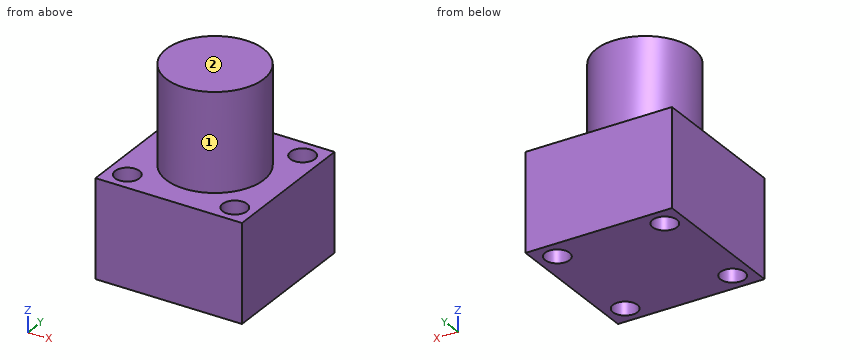
Autodesk Inventor part; units mm, degrees
ref_plane "YZ Plane" through (0, 0, 0) normal (1, 0, 0) x (0, 1, 0)
ref_plane "XZ Plane" through (0, 0, 0) normal (0, 1, 0) x (-1, 0, 0)
ref_plane "XY Plane" through (0, 0, 0) normal (0, 0, 1) x (1, 0, 0)
sketch "Sketch1" plane through (0, 0, 0) normal (0, 0, 1) x (1, 0, 0)
  line L0 (-6.0176, 0) -> (13.0324, 0)
  line L1 (13.0324, 0) -> (13.0324, 19.05)
  line L2 (13.0324, 19.05) -> (-6.0176, 19.05)
  line L3 (-6.0176, 19.05) -> (-6.0176, 0)
  point P0 (0, 0)
  dimension "d0" = 19.05
  dimension "d1" = 19.05
extrude "Extrusion1" add sketch "Sketch1" along normal blind 12.7
sketch "Sketch2" plane through (0, 0, 12.7) normal (0, 0, 1) x (1, 0, 0)
  circle A0 centre (3.5074, 9.525) radius 6.35
  line L0 (13.0324, 19.05) -> (-6.0176, 19.05)
  line L1 (13.0324, 0) -> (13.0324, 19.05)
  circle A1 centre (10.4924, 16.51) radius 1.5875
  circle A2 centre (10.4924, 2.54) radius 1.5875
  line L2 (-6.0176, 0) -> (13.0324, 0)
  circle A3 centre (-3.4776, 16.51) radius 1.5875
  line L3 (-6.0176, 19.05) -> (-6.0176, 0)
  circle A4 centre (-3.4776, 2.54) radius 1.5875
  point P0 (0, 0)
  dimension "d4" = 9.525
  dimension "d5" = 9.525
  dimension "d6" = 12.7
  dimension "d9" = 3.175
  dimension "d10" = 2.54
  dimension "d11" = 2.54
  dimension "d12" = 3.175
  dimension "d13" = 2.54
  dimension "d14" = 2.54
  dimension "d15" = 3.175
  dimension "d16" = 2.54
  dimension "d17" = 2.54
  dimension "d18" = 3.175
  dimension "d19" = 2.54
  dimension "d20" = 2.54
extrude "Extrusion2" add sketch "Sketch2" along normal blind 12.7 contours A0
sketch "Sketch3" plane through (0, 0, 12.7) normal (0, 0, 1) x (1, 0, 0)
  circle A0 centre (10.4924, 16.51) radius 1.5875
  circle A1 centre (-3.4776, 16.51) radius 1.5875
  circle A2 centre (-3.4776, 2.54) radius 1.5875
  circle A3 centre (10.4924, 2.54) radius 1.5875
  line L0 (-6.0176, 0) -> (13.0324, 0)
  line L1 (-6.0176, 19.05) -> (-6.0176, 0)
  line L2 (13.0324, 19.05) -> (-6.0176, 19.05)
  line L3 (13.0324, 0) -> (13.0324, 19.05)
  point P0 (0, 0)
  dimension "d21" = 3.175
  dimension "d22" = 3.175
  dimension "d23" = 3.175
  dimension "d24" = 3.175
  dimension "d25" = 2.54
  dimension "d26" = 2.54
  dimension "d27" = 2.54
  dimension "d28" = 2.54
  dimension "d29" = 2.54
  dimension "d30" = 2.54
  dimension "d31" = 2.54
  dimension "d32" = 2.54
extrude "Extrusion3" cut sketch "Sketch3" against normal blind 12.7 contours A0 | A1 | A2 | A3
properties part number "bottom piece pvc"
CAD build for the part. Positions are in the model's coordinates, mm. Face numbers are marked on the shaded views. A direction names the side the tool comes from. Coordinates: 2 decimals unless noted, no trailing zeros. Write each loop counter-clockwise with the first axis right and the second up, starting at its lowest first coordinate (ties: lowest second). Pieces come first, ordered by that corner, then holes. Notation, with made-up numbers: (89, -7.75) -> (141, -7.75) arc R37 ccw to (141, 28.25) -> close; hole circle Ø8 at (33.5, 79). An arc over 180 degrees is marked (long way). Use CSV: the item, a comma, the result in double quotes. Start each with the question number.
Item 1: Drop flat-ended pins along their axis: P1, Ø8, axis at x = 8.5, z = 19.5, coming from the +Y side; P2, Ø3.5, axis at x = -3.48, y = 2.54, coming from the +Z side; P3, Ø1, axis at y = 9.5, z = 22.5, coming from the +X side. Give the stop position or say it passes through.
Item 2: Band-saw the part on B-B, the plane x = -3.25. Write the cut outline in (y, z), plus the area to 3 significant figures.
Item 3: Tool access for the marked faces 1 and 2: list every direction of +Z, -Z, +X, -X, +Y, -Y with a clear straight run to the whole face (end or side of a thin tool).
Item 4: Wall check: probe 1 along X at (y, z) = (3, 9); probe 2 along Y at (x, z) = (10, 7); probe 3 along Z at (x, y) = (8.75, 18.25). Give the ranges that are in metal, low to high.
Item 5: Band-saw the part on A-A, the plane z = 2.5. Give the number of separate pieces and of enclosed holes in the cut face, plus the area to 3 significant figures.
Item 6: Band-saw the part on C-C, the plane y = 16.51. Write the cut outline in (x, z).
Item 7: Band-saw the part on D-D, the plane y = 11.5. Write the cut outline in (x, z).
Response values:
1,P1,"stops at y = 15.8"
1,P2,"stops at z = 12.7"
1,P3,"stops at x = 9.86"
2,outline,"(0, 0) -> (0.97, 0) -> (0.97, 12.7) -> (0, 12.7) -> close; (4.11, 0) -> (14.94, 0) -> (14.94, 12.7) -> (4.11, 12.7) -> close; (18.08, 0) -> (19.05, 0) -> (19.05, 12.7) -> (18.08, 12.7) -> close"
2,area,"162 mm2"
3,face 1,"+Z"
3,face 2,"+Z, +X, -X, +Y, -Y"
4,probe 1,"x = -6.02 to -5, -1.96 to 8.97, 12.01 to 13.03"
4,probe 2,"y = 0 to 1.03, 4.05 to 15, 18.02 to 19.05"
4,probe 3,"z = 0 to 12.7"
5,separate pieces,"1"
5,enclosed holes,"4"
5,area,"331 mm2"
6,outline,"(-6.02, 0) -> (-5.07, 0) -> (-5.07, 12.7) -> (-6.02, 12.7) -> close; (-1.89, 0) -> (8.9, 0) -> (8.9, 12.7) -> (-1.89, 12.7) -> close; (12.08, 0) -> (13.03, 0) -> (13.03, 12.7) -> (12.08, 12.7) -> close"
7,outline,"(-6.02, 0) -> (13.03, 0) -> (13.03, 12.7) -> (9.54, 12.7) -> (9.54, 25.4) -> (-2.53, 25.4) -> (-2.53, 12.7) -> (-6.02, 12.7) -> close"
